The model under review builds one solid part; all positions refer to its coordinate system, in mm. Face numbers are marked on the shaded views. A direction names the side the tool comes from. Round coordinates to 2 decimals unless told otherwise and drop trailing zeros. Loops run counter-clockwise (first coordinate to the right, second up) from the corner with the lowest first, then second, coordinate; pieces in that order, holes last. Notation, with made-up numbers: M -4,-24 L 17,-24 A13 cw 17,-13 Z; hole C -32,31 d11. An arc over 180 degrees is marked long. Use a Markdown table: item, result. Add a question column.
```python
from build123d import *

# Parameters (mm, degrees)
BOSS_EXTRUDE1_DEPTH = 5.8
FILLET1_R           = 0.05
FILLET2_R           = 0.2
SKETCH2_R           = 1.35
SKETCH2_R_2         = 1
BOSS_EXTRUDE2_DEPTH = 2


with BuildPart() as part:
    # Sketch1 → Boss-Extrude1 (new body)
    with BuildSketch(Plane(origin=(0, 0, 0), x_dir=(1, 0, 0), z_dir=(0, 1, 0))):
        with BuildLine():
            Line((-0.448807004, -1.058807004), (-0.106066017, -0.716066017))
            ThreePointArc((-0.106066017, -0.716066017), (0, -0.672132034), (0.106066017, -0.716066017))
            Line((0.106066017, -0.716066017), (0.448807004, -1.058807004))
            ThreePointArc((0.448807004, -1.058807004), (0, 1.15), (-0.448807004, -1.058807004))
        make_face()
        with BuildLine():
            Line((-0.479612457, -0.877480422), (-0.212132034, -0.61))
            ThreePointArc((-0.212132034, -0.61), (0, -0.522132034), (0.212132034, -0.61))
            Line((0.212132034, -0.61), (0.479612457, -0.877480422))
            ThreePointArc((0.479612457, -0.877480422), (0, 1), (-0.479612457, -0.877480422))
        make_face(mode=Mode.SUBTRACT)
    extrude(amount=BOSS_EXTRUDE1_DEPTH)

    # Fillet1
    fillet1_edges = [part.edges().sort_by_distance(p)[0] for p in [
        (0.479612457, 2.9, 0.877480422),
        (-0.479612457, 2.9, 0.877480422),
    ]]
    fillet(fillet1_edges, radius=FILLET1_R)

    # Fillet2
    fillet2_edges = [part.edges().sort_by_distance(p)[0] for p in [
        (-0.448807004, 2.9, 1.058807004),
        (0.448807004, 2.9, 1.058807004),
    ]]
    fillet(fillet2_edges, radius=FILLET2_R)

    # Sketch2 → Boss-Extrude2 (add)
    with BuildSketch(Plane(origin=(0, 5.8, 0), x_dir=(1, 0, 0), z_dir=(0, 1, 0))):
        Circle(SKETCH2_R)
        Circle(SKETCH2_R_2, mode=Mode.SUBTRACT)
    extrude(amount=BOSS_EXTRUDE2_DEPTH)


solid = part.part
```
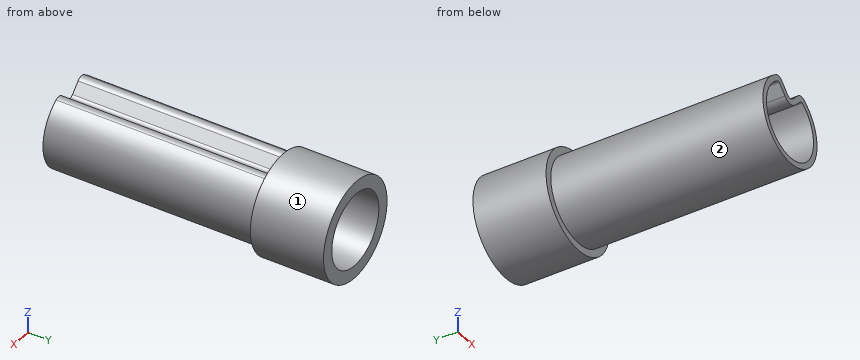
(1) For the marked faces 1 and 2, list the 3-axis set-ups (+Z, -Z, +X, -X, +Y, -Y) from which the entire face can be reached by the end or side of a thin tool; tool diameter is ignored.
(2) Consider section C-C, the plane x = 0. Give the boundary of the cut face in (y, z).
(3) Consider section A-A, the plane y = 4.75. Give the boundary of the cut face in (x, z).
(4) Insertion check: pin 1 Ø1 at (x, y) = (-0.5, 2.5) entering from -Z. The pin has a flat end and moves straight along its axis. Give the tip position at first contact, or say it passes through.
(5) Consider section D-D, the plane x = -0.8. Give the boundary of the cut face in (y, z), then the cut area to 3 significant figures.
(6) To check wall thickness, follow probe 1 along Z at (x, y) = (0, 6.2); probe 2 along X at (y, z) = (3.75, 0.6). State the ranges of each line that lie inside material, in increasing order.
(7) Consider section B-B, the plane z = 0. Give the boundary of the cut face in (x, y).
Found:
| question | item | result |
|---|---|---|
| 1 | face 1 | +Y, -Y |
| 1 | face 2 | -Y |
| 2 | outline | M 0,-1.15 L 5.8,-1.15 L 5.8,-1.35 L 7.8,-1.35 L 7.8,-1 L 0,-1 Z; M 0,0.52 L 5.8,0.52 L 5.8,0.67 L 0,0.67 Z; M 5.8,1 L 7.8,1 L 7.8,1.35 L 5.8,1.35 Z |
| 3 | outline | M -0.59,0.99 A1.15 ccw long 0.59,0.99 A0.2 ccw 0.35,0.96 L 0.11,0.72 A0.15 cw -0.11,0.72 L -0.35,0.96 A0.2 ccw Z; hole M -0.51,0.86 A1 ccw long 0.51,0.86 A0.05 ccw 0.45,0.85 L 0.21,0.61 A0.3 cw -0.21,0.61 L -0.45,0.85 A0.05 ccw Z |
| 4 | pin 1 | stops at z = -1.15 |
| 5 | outline | M 0,-0.83 L 5.8,-0.83 L 5.8,-1.09 L 7.8,-1.09 L 7.8,-0.6 L 0,-0.6 Z; M 0,0.6 L 7.8,0.6 L 7.8,1.09 L 5.8,1.09 L 5.8,0.83 L 0,0.83 Z |
| 5 | area | 4.57 mm^2 |
| 6 | probe 1 | z = -1.35 to -1, 1 to 1.35 |
| 6 | probe 2 | x = -0.98 to -0.8, -0.2 to 0.2, 0.8 to 0.98 |
| 7 | outline | M -1.35,5.8 L -1.15,5.8 L -1.15,0 L -1,0 L -1,7.8 L -1.35,7.8 Z; M 1,0 L 1.15,0 L 1.15,5.8 L 1.35,5.8 L 1.35,7.8 L 1,7.8 Z |
